Autodesk Inventor part; units mm, degrees
ref_plane "ANBAU_XY" through (0, 0, 0) normal (0, 0, -1) x (1, 0, 0)
ref_plane "ANBAU_YZ" through (0, 0, 0) normal (1, 0, 0) x (0, -1, 0)
ref_plane "ANBAU_ZX" through (0, 0, 0) normal (0, -1, 0) x (0, 0, -1)
sketch "Sketch_3" plane through (0, 0, 0) normal (1, 0, 0) x (0, 1, 0)
  line L0 (0, 0) -> (0, 86)
  line L1 (0, 86) -> (2.3865, 86)
  line L2 (2.3865, 86) -> (3, 85.3865)
  line L3 (3, 85.3865) -> (3, 73.2685)
  line L4 (3, 73.2685) -> (2.4, 71.62)
  line L5 (2.4, 71.62) -> (2.4, 70.4)
  arc A0 (2.4, 70.4) -> (2.8, 70) centre (2.8, 70.4) ccw
  line L6 (2.8, 70) -> (3, 69.8)
  line L7 (3, 69.8) -> (3, 10)
  line L8 (3, 10) -> (6, 10)
  line L9 (6, 10) -> (6, 0)
  line L10 (6, 0) -> (0, 0)
  line L11 (0, 0) -> (0, 86)
revolve "Revolution1" add sketch "Sketch_3" angle 360 about axis through (0, 0, 0) along (0, 0, -1)
thread "Thread1"
sketch "Sketch_4" plane through (0, 0, 0) normal (0, 1, 0) x (-1, 0, 0)
  line L0 (5, 65.5566) -> (5, 71)
  line L1 (5, 71) -> (2.5, 71)
  line L2 (2.5, 71) -> (2.5, 67)
  line L3 (2.5, 67) -> (5, 65.5566)
extrude "Extrusion1" cut sketch "Sketch_4" along normal mid plane 6
sketch "Sketch_5" plane through (0, 0, 0) normal (0, 1, 0) x (-1, 0, 0)
  line L0 (-2.5, 67) -> (-2.5, 71)
  line L1 (-2.5, 71) -> (-5, 71)
  line L2 (-5, 71) -> (-5, 65.5566)
  line L3 (-5, 65.5566) -> (-2.5, 67)
extrude "Extrusion2" cut sketch "Sketch_5" along normal mid plane 6
ref_plane "ANBAU_XY" through (0, 0, 0) normal (0, 0, -1) x (1, 0, 0)
ref_plane "ANBAU_YZ" through (0, 0, 0) normal (1, 0, 0) x (0, -1, 0)
ref_plane "ANBAU_ZX" through (0, 0, 0) normal (0, -1, 0) x (0, 0, -1)
ref_plane "FDT_KSAUFSATZ_XY" through (0, 0, 76.2) normal (0, 0, 1) x (1, 0, 0)
ref_plane "FDT_KSAUFSATZ_YZ" through (0, 0, 76.2) normal (1, 0, 0) x (0, 1, 0)
ref_plane "FDT_KSAUFSATZ_ZX" through (0, 0, 76.2) normal (0, 1, 0) x (0, 0, 1)
ref_plane "FDT_NUT_XY" through (0, 0, 76.2) normal (0, 0, 1) x (1, 0, 0)
ref_plane "FDT_NUT_YZ" through (0, 0, 76.2) normal (1, 0, 0) x (0, 1, 0)
ref_plane "FDT_NUT_ZX" through (0, 0, 76.2) normal (0, 1, 0) x (0, 0, 1)
ref_plane "to_nut_XY" through (0, 0, 83.325) normal (0, 0, 1) x (1, 0, 0)
ref_plane "to_nut_YZ" through (0, 0, 83.325) normal (1, 0, 0) x (0, 1, 0)
ref_plane "to_nut_ZX" through (0, 0, 83.325) normal (0, 1, 0) x (0, 0, 1)
properties part number "8112003 DSNU-S-12-30-P---(P)"
Geometry: final body of the model. Coordinates: model frame, mm. A direction names the side the tool comes from. Give positions to 0.01 mm unless a question says otherwise; leave off trailing zeros. Write each loop counter-clockwise with the first axis right and the second up, starting at its lowest first coordinate (ties: lowest second). Pieces come first, ordered by that corner, then holes.
(1) Cut plane B-B, the plane x = 0. Return loops of the section in (y, z).
(2) Access query for faces 5 (the flat face through (-2.5, 0, 69)), 6 (the cylindrical face through (2.024, 1.29, 71.001)), 7 (the cylindrical face through (0, -3, 79)). Directions: +Z, -Z, +X, -X, +Y, -Y. A direction counts if a zero-diameter tool reaches every point of the face in a straight line with its end or side. Return the directions, or none.
(3) Mould query, pull axis Z, two halves, no side actions, for faces 1 (the flat face through (0, 0, 86)), 2 (the cylindrical face through (0, -6, 5)), 3 (the flat face through (2.5, 0, 69)), 4 (the flat face through (0, 0, 0)). Classes: released by +Z, released by -Z, zero draft, split by the parting line, or undercut.
(4) Ray query, line 1 (Z direction, x = 3, y = -4.5); line 2 (X direction, y = -2.5, z = 73.5); line 3 (Y direction, x = -1.5, z = 25.5). Return the intervals inside material, ascending.
(5) Cut plane D-D, the plane x = 5.25. Return loops of the section in (y, z), then the cut area to 3 significant figures.
(6) Cut plane A-A, the plane y = 0. Return loops of the section in (x, z).
(7) First-contact query: P1, Ø2, axis at x = -4, y = -1, coming from the +Z side; P2, Ø2, axis at x = -4.5, z = 12.5, coming from the +Y side; P3, Ø6, axis at x = 0, z = 22.5, coming from the -Y side; P4, Ø4, axis at y = 2.5, z = 41, coming from the +X side. Flat tips, straight axial feed; report the tip coordinate or a pass-through.
(8) Cut plane C-C, the plane z = 14. Return loops of the section in (x, y).
Values follow:
1. outline: (-6, 0) - (6, 0) - (6, 10) - (3, 10) - (3, 69.8) - (2.8, 70) arc R0.4 cw to (2.4, 70.4) - (2.4, 71.62) - (3, 73.27) - (3, 85.39) - (2.39, 86) - (-2.39, 86) - (-3, 85.39) - (-3, 73.27) - (-2.4, 71.62) - (-2.4, 70.4) arc R0.4 cw to (-2.8, 70) - (-3, 69.8) - (-3, 10) - (-6, 10) - close
2. face 5: -X, +Y, -Y
2. face 6: none
2. face 7: +Z
3. face 1: released by +Z
3. face 2: zero draft
3. face 3: undercut
3. face 4: released by -Z
4. line 1: z = 0 to 10
4. line 2: x = -1.66 to 1.66
4. line 3: y = -2.6 to 2.6
5. outline: (-2.9, 0) - (2.9, 0) - (2.9, 10) - (-2.9, 10) - close
5. area: 58.1 mm2
6. outline: (-6, 0) - (6, 0) - (6, 10) - (3, 10) - (3, 66.71) - (2.5, 67) - (2.5, 70.14) arc R0.4 cw to (2.4, 70.4) - (2.4, 71.62) - (3, 73.27) - (3, 85.39) - (2.39, 86) - (-2.39, 86) - (-3, 85.39) - (-3, 73.27) - (-2.4, 71.62) - (-2.4, 70.4) arc R0.4 cw to (-2.5, 70.14) - (-2.5, 67) - (-3, 66.71) - (-3, 10) - (-6, 10) - close
7. P1: stops at z = 10
7. P2: passes through
7. P3: stops at y = -3
7. P4: stops at x = 2.96
8. outline: circle Ø6 at (0, 0)
